from build123d import *

# Parameters (mm, degrees)
F0_W      = 100
F0_H      = 80
F1_DEPTH  = 45
F5_DEPTH  = 45
F6_R      = 7.5
F8_DEPTH  = 30
F9_DEPTH  = 20
F3_W      = 20
F3_H      = 10
F10_DEPTH = 15
F12_DEPTH = 80


with BuildPart() as f1:
    # F0 (on Top) → F1 (new body)
    with BuildSketch(Plane.XY):
        with Locations((-1.529125, 6.107334)):
            Rectangle(F0_W, F0_H)
    extrude(amount=F1_DEPTH)

    # F4 (on face) → F5 (cut)
    with BuildSketch(Plane.XY.offset(45)):
        with BuildLine():
            ThreePointArc((11.716428, -3.892666), (-0.075549, 13.568155), (-16.529125, 26.729113))
            Line((-16.529125, 26.729113), (-16.529125, -3.892666))
            Line((-16.529125, -3.892666), (11.716428, -3.892666))
        make_face()
    extrude(amount=-F5_DEPTH, mode=Mode.SUBTRACT)

    # F6 (on face) → F8 (cut, through all)
    with BuildSketch(Plane.XY.offset(45)):
        with Locations((8.470875, 31.107334)):
            Circle(F6_R)
    extrude(amount=-F8_DEPTH, mode=Mode.SUBTRACT)

    # F4 (on face) → F9 (cut)
    with BuildSketch(Plane.XY.offset(45)):
        with BuildLine():
            Line((-16.529125, -3.892666), (-16.529125, 26.729113))
            ThreePointArc((-16.529125, 26.729113), (-33.411792, 33.722142), (-51.529125, 36.107334))
            Line((-51.529125, 36.107334), (-51.529125, -33.892666))
            Line((-51.529125, -33.892666), (18.470875, -33.892666))
            ThreePointArc((18.470875, -33.892666), (16.761389, -18.517177), (11.716428, -3.892666))
            Line((11.716428, -3.892666), (-16.529125, -3.892666))
        make_face()
    extrude(amount=-F9_DEPTH, mode=Mode.SUBTRACT)

    # F3 (on face) → F10 (join)
    with BuildSketch(Plane.XZ.offset(33.892666)):
        with Locations((-41.529125, 30)):
            Rectangle(F3_W, F3_H)
    extrude(amount=-F10_DEPTH)

    # F11 (on face) → F12 (cut, through all)
    with BuildSketch(Plane.XZ.offset(33.892666)):
        with BuildLine():
            ThreePointArc((32.089901, 45), (44.248271, 23.944395), (48.470875, 0))
            Line((48.470875, 0), (48.470875, 45))
            Line((48.470875, 45), (32.089901, 45))
        make_face()
    extrude(amount=-F12_DEPTH, mode=Mode.SUBTRACT)


solid = f1.part
Geometry check sheet. Reference: the model listing, model coordinates, mm. A direction names the side the tool comes from. Coordinates: 2 decimals unless noted, no trailing zeros. Order: outer loops, then holes, each group sorted by start corner. A loop starts at its lowest first (then second) coordinate and runs counter-clockwise, first axis right, second up. Notation, with made-up numbers: (-31.5, 29) - (23.5, 29) arc R11 ccw to (23.5, 36) - close; hole circle Ø7 at (33, 52.5). An arc over 180 degrees is marked (long way). Answer in a Markdown table with one row per item. Add a question column.
1) Cross-section at D-D, the plane y = 8. Record the cut outline in (x, z), then the cut area to 3 significant figures.
2) Release check for a two-part mould opening along Y. For faces 1 (the flat face through (-42, -26, 35)), 2 (the flat face through (-2, -33.893, 18)), 3 (the flat face through (-16.529, 12, 13)) record: +Y half, -Y half, draft (parallel to the pull), parting line (faces both ways), or undercut.
3) Material ranges on line 1 along Z through (x, y) = (-17, -14); line 2 along X through (y, z) = (20, 5); line 3 along X through (y, z) = (29, 32.5), recorded low to high. Write a range as [from, to].
4) Cross-section at A-A, the plane z = 32. Record the cut outline in (x, y).
5) Gauge pin test, flat ends, axial feed: P1, Ø12, axis at x = 8, y = 30, coming from the +Z side; P2, Ø2, axis at y = 36, z = 21, coming from the +X side; P3, Ø7.5, axis at x = -46, y = -23, coming from the +Z side. Record the tip position at first contact, or that the pin passes through.
6) Set-up check for faces 4 (the flat face through (8, 31, 15)), 5 (the flat face through (-3, -3.893, 13)), 6 (the flat face through (-42, -18.893, 30)): record each of +Z, -Z, +X, -X, +Y, -Y from which the full face is reachable in a straight line by a thin tool's end or side.
7) Cross-section at B-B, the plane x = 5. Record the cut outline in (y, z), then the cut area to 3 significant figures.
8) Cross-section at C-C, the plane z = 22. Record the cut outline in (x, y).
Check result:
| question | item | result |
|---|---|---|
| 1 | outline | (-51.53, 0) - (-16.53, 0) - (-16.53, 25) - (-51.53, 25) - close; (4.55, 0) - (48.47, 0) arc R70 ccw to (32.09, 45) - (4.55, 45) - close |
| 1 | area | 2,620 mm² |
| 2 | face 1 | draft |
| 2 | face 2 | -Y half |
| 2 | face 3 | undercut |
| 3 | line 1 | z = [0, 25] |
| 3 | line 2 | x = [-51.53, -16.53], [-6.86, 48.29] |
| 3 | line 3 | x = [-20.8, 1.27], [15.67, 40.47] |
| 4 | outline | (-51.53, -33.89) - (-31.53, -33.89) - (-31.53, -18.89) - (-51.53, -18.89) - close; (-51.53, 36.11) arc R70 cw to (-16.53, 26.73) arc R70 cw to (11.72, -3.89) arc R70 cw to (18.47, -33.89) - (40.73, -33.89) - (40.73, 46.11) - (-51.53, 46.11) - close; hole circle Ø15 at (8.47, 31.11) |
| 5 | P1 | stops at z = 15 |
| 5 | P2 | stops at x = 45.55 |
| 5 | P3 | stops at z = 35 |
| 6 | face 4 | +Z |
| 6 | face 5 | +Z, -Z |
| 6 | face 6 | +Z, -X |
| 7 | outline | (-33.89, 0) - (-3.89, 0) - (-3.89, 25) - (-33.89, 25) - close; (7.39, 0) - (46.11, 0) - (46.11, 45) - (37.76, 45) - (37.76, 15) - (24.46, 15) - (24.46, 45) - (7.39, 45) - close |
| 7 | area | 2,090 mm² |
| 8 | outline | (-51.53, -33.89) - (44.92, -33.89) - (44.92, 46.11) - (-51.53, 46.11) - close; hole (-16.53, -3.89) - (11.72, -3.89) arc R70 ccw to (-16.53, 26.73) - close; hole circle Ø15 at (8.47, 31.11) |
